Read the model definition and answer for the solid it produces. Units are mm, in the model's axes. A direction names the side the tool comes from. Round coordinates to 2 decimals unless told otherwise and drop trailing zeros. Order: outer loops, then holes, each group sorted by start corner. A loop starts at its lowest first (then second) coordinate and runs counter-clockwise, first axis right, second up. Notation, with made-up numbers: (-13, 28.25) -> (9, 28.25) arc R26 ccw to (9, 62.25) -> close; hole circle Ø7 at (4.5, -33). An arc over 180 degrees is marked (long way). One line per item, written item: value. Start each with the question number.
1. Consider line 1 (X direction, y = 1.5, z = 8); line 2 (Y direction, x = -1.5, z = 7.75); line 3 (Y direction, x = 39.8, z = 15). Determine where each line is inside the solid, lowest interval first.
2. Section B-B (z = 3) is taken. Give the vertices of the cut face in (x, y).
3. Section A-A (y = 1.5) is taken. Give the vertices of the cut face in (x, z), then the cut area to 3 significant figures.
4. Section C-C (z = 17.5) is taken. Give the vertices of the cut face in (x, y), then the cut area to 3 significant figures.
5. Flat-ended cylindrical pins translate along their axes: pin 1 Ø14.5 at (x, y) = (-8, 3.5) entering from +Z; pin 2 Ø6 at (x, y) = (1.5, 11) entering from -Z; pin 3 Ø7.5 at (y, z) = (15.12, 15) entering from +X; pin 4 Ø9.5 at (y, z) = (-15.23, 13.88) entering from -X. Find the tip coordinate at first contact, or state that the pin passes through.
6. For faces 1 (the face through (39.507, 11.09, 12.905)), 2 (the face through (-0.2, 24.2, 30)), 3 (the face through (-1, 0, 0)), 4 (the face through (-39.507, -14.188, 21.813)), 5 (the face through (-1, 24, 15)), determine the directions among +Z, -Z, +X, -X, +Y, -Y from which every point of the face is accessible in a straight line to the end or side of a thin tool.
7. The mould has two halves that part along X. Classify faces 6 (the face through (-40, 0, 15)), 7 (the face through (40, 0, 15)), 8 (the face through (-1, 25, 15)), 9 (the face through (-39, 5, 15)): released by +X, released by -X, zero draft, split by the parting line, or undercut.
8. Section D-D (x = -3.5) is taken. Give the vertices of the cut face in (y, z), then the cut area to 3 significant figures.
from build123d import *

# Parameters (mm, degrees)
SKETCH_1_W          = 80
SKETCH_1_H          = 50
EXTRUDE_1_DEPTH     = 30
SHELL_1_T           = -1
SKETCH_3_R          = 4.539465833
CUT_EXTRUDE_1_DEPTH = 30
SKETCH_4_R          = 8
CUT_EXTRUDE_2_DEPTH = 30


with BuildPart() as part:
    # 草图1 → 凸台-拉伸1 (new body)
    with BuildSketch(Plane.XY):
        Rectangle(SKETCH_1_W, SKETCH_1_H)
    extrude(amount=EXTRUDE_1_DEPTH)

    # 抽壳1
    shell_1_openings = [part.faces().sort_by_distance(p)[0] for p in [
        (0, 0, 30),
    ]]
    offset(amount=SHELL_1_T, openings=shell_1_openings, kind=Kind.INTERSECTION)

    # 草图3 → 切除-拉伸1 (cut)
    with BuildSketch(Plane(origin=(40, 0, 0), x_dir=(0, 0, -1), z_dir=(1, 0, 0))):
        with Locations((-15, 15.117251004)):
            Circle(SKETCH_3_R)
    extrude(amount=-CUT_EXTRUDE_1_DEPTH, mode=Mode.SUBTRACT)

    # 草图4 → 切除-拉伸2 (cut)
    with BuildSketch(Plane.ZY.offset(40)):
        with Locations(Location((13.881500003, -15.22906305, 0), (0, 0, 270))):
            Circle(SKETCH_4_R)
    extrude(amount=-CUT_EXTRUDE_2_DEPTH, mode=Mode.SUBTRACT)


solid = part.part
Answer:
1. line 1: -40 to -39, 39 to 40
1. line 2: -25 to -24, 24 to 25
1. line 3: -25 to 10.58, 19.66 to 25
2. outline: (-40, -25) -> (40, -25) -> (40, 25) -> (-40, 25) -> close; hole (-39, -24) -> (39, -24) -> (39, 24) -> (-39, 24) -> close
3. outline: (-40, 0) -> (40, 0) -> (40, 30) -> (39, 30) -> (39, 1) -> (-39, 1) -> (-39, 30) -> (-40, 30) -> close
3. area: 138 mm^2
4. outline: (-40, -25) -> (40, -25) -> (40, 11.33) -> (39, 11.33) -> (39, -24) -> (-39, -24) -> (-39, -22.36) -> (-40, -22.36) -> close; (-40, -8.09) -> (-39, -8.09) -> (-39, 24) -> (39, 24) -> (39, 18.91) -> (40, 18.91) -> (40, 25) -> (-40, 25) -> close
4. area: 234 mm^2
5. pin 1: z = 1
5. pin 2: z = 0
5. pin 3: x = -39
5. pin 4: x = 39
6. face 1: +X
6. face 2: +Z, +X, -X, +Y, -Y
6. face 3: -Z, +X, -X, +Y, -Y
6. face 4: -X
6. face 5: +Z
7. face 6: released by -X
7. face 7: released by +X
7. face 8: zero draft
7. face 9: undercut
8. outline: (-25, 0) -> (25, 0) -> (25, 30) -> (24, 30) -> (24, 1) -> (-24, 1) -> (-24, 30) -> (-25, 30) -> close
8. area: 108 mm^2
